Work out the finished part from the listing and answer in its coordinate system (mm). A direction names the side the tool comes from. Coordinates: 2 decimals unless noted, no trailing zeros. Order: outer loops, then holes, each group sorted by start corner. A loop starts at its lowest first (then second) coordinate and runs counter-clockwise, first axis right, second up. Notation, with made-up numbers: (19, 52.5) -> (67, 52.5) arc R15 ccw to (67, 68.5) -> close; hole circle Ø8 at (57.25, 78). An arc over 180 degrees is marked (long way). Write item = value, one per line. Start each with the question number.
Q1. For a pull along Z with two mould halves and no side action, classify faces 1 (the flat face through (3, -3.057, 3)), 2 (the flat face through (3, -15, 20)), 3 (the flat face through (3, -7, 7)), 4 (the flat face through (3, -4, -10)) as +Z half, -Z half, draft (parallel to the pull), parting line (faces both ways), or undercut.
Q2. Flat-ended cylindrical pins translate along their axes: pin 1 (1.2 mm diameter, centred on x = 2, y = -4.5, fed in from +Z); pin 2 (1.7 mm diameter, centred on x = 3, y = 3.5, fed in from +Z); pin 3 (1.7 mm diameter, centred on x = 2, z = 25, fed in from -Y); pin 4 (1.1 mm diameter, centred on x = 2, z = 3.5, fed in from +Y). Find the tip coordinate at first contact, or state that the pin passes through.
Q3. Which of the six approach directions +Z, -Z, +X, -X, +Y, -Y give full straight-line access (tool end or side, diameter ignored) to faces 5 (the flat face through (3, 12, -7)), 6 (the flat face through (3, -10, 25)), 7 (the flat face through (3, -6, 10.031)), 8 (the flat face through (3, 6, -3.969)), 9 (the flat face through (5.6, -11, 5))?
Q4. The part is cut by section C-C, the plane y = -11.5. Determine the outline of the cut face in (x, z).
Q5. The part is cut by section A-A, the plane x = 3.65. Determine the outline of the cut face in (y, z), plus the area to 3 significant figures.
Q6. Straight lines are drawn through the part: L1, parallel to Z at x = 4.25, y = -6; L2, parallel to Y at x = 4.6, z = 18; L3, parallel to Y at x = 3.5, z = 24. For each, find the intervals that lie inside material, in ascending order. Write a range as from..to.
Q7. The part is cut by section B-B, the plane z = 21. Determine the outline of the cut face in (x, y).
```python
from build123d import *

# Parameters (mm, degrees)
BOSS_EXTRUDE1_DEPTH = 5.6


with BuildPart() as part:
    # Sketch1 → Boss-Extrude1 (new body)
    with BuildSketch(Plane(origin=(0, 0, 0), x_dir=(0, 0, -1), z_dir=(1, 0, 0))):
        with BuildLine():
            Line((3.96875, 0), (3.96875, 12))
            Line((3.96875, 12), (10, 12))
            Line((10, 12), (10, -20))
            Line((10, -20), (-20, -20))
            Line((-20, -20), (-20, -10))
            Line((-20, -10), (-30, -10))
            Line((-30, -10), (-30, -5))
            Line((-30, -5), (-10.03125, -5))
            Line((-10.03125, -5), (-10.03125, -7))
            Line((-10.03125, -7), (-3.53125, -7))
            Line((-3.53125, -7), (-3.53125, -3.056754815))
            Line((-3.53125, -3.056754815), (-2.53125, -3.056754815))
            ThreePointArc((-2.53125, -3.056754815), (1.68894614, -3.591439475), (3.96875, 0))
        make_face()
    extrude(amount=BOSS_EXTRUDE1_DEPTH)


solid = part.part
```
Model answer:
q1.face_1 = draft
q1.face_2 = +Z half
q1.face_3 = undercut
q1.face_4 = -Z half
q2.pin_1 = 30
q2.pin_2 = -3.97
q2.pin_3 = -10
q2.pin_4 = -3.06
q3.face_5 = +Z, -Z, +X, -X, +Y
q3.face_6 = +Z, +X, -X, -Y
q3.face_7 = +X, -X, +Y
q3.face_8 = +Z, +X, -X, +Y
q3.face_9 = +Z, -Z, +X, +Y, -Y
q4.outline = (0, -10) -> (5.6, -10) -> (5.6, 20) -> (0, 20) -> close
q5.outline = (-20, -10) -> (12, -10) -> (12, -3.97) -> (0, -3.97) arc R3.97 cw to (-3.06, 2.53) -> (-3.06, 3.53) -> (-7, 3.53) -> (-7, 10.03) -> (-5, 10.03) -> (-5, 30) -> (-10, 30) -> (-10, 20) -> (-20, 20) -> close
q5.area = 602 mm2
q6.L1 = -10..3.53, 10.03..30
q6.L2 = -20..-5
q6.L3 = -10..-5
q7.outline = (0, -10) -> (5.6, -10) -> (5.6, -5) -> (0, -5) -> close
